Source: CAD feature listing. Evaluate the final solid. Frame: model axes, mm. A direction names the side the tool comes from. Coordinates: 2 decimals unless noted, no trailing zeros. Order: outer loops, then holes, each group sorted by start corner. A loop starts at its lowest first (then second) coordinate and runs counter-clockwise, first axis right, second up.
```python
from build123d import *

# Parameters (mm, degrees)
SKETCH1_W           = 42
SKETCH1_H           = 42
BOSS_EXTRUDE1_DEPTH = 46
CHAMFER1_SIZE       = 5
SKETCH2_R           = 11.5
BOSS_EXTRUDE2_DEPTH = 2
SKETCH3_R           = 2.5
BOSS_EXTRUDE3_DEPTH = 25
SKETCH4_R           = 1.5
CUT_EXTRUDE1_DEPTH  = 5


with BuildPart() as part:
    # Sketch1 → Boss-Extrude1 (new body)
    with BuildSketch(Plane(origin=(0, 0, 0), x_dir=(1, 0, 0), z_dir=(0, 1, 0))):
        Rectangle(SKETCH1_W, SKETCH1_H)
    extrude(amount=BOSS_EXTRUDE1_DEPTH)

    # Chamfer1
    chamfer1_edges = [part.edges().sort_by_distance(p)[0] for p in [
        (21, 23, 21),
        (-21, 23, 21),
        (-21, 23, -21),
        (21, 23, -21),
    ]]
    chamfer(chamfer1_edges, length=CHAMFER1_SIZE)

    # Sketch2 → Boss-Extrude2 (add)
    with BuildSketch(Plane(origin=(0, 46, 0), x_dir=(1, 0, 0), z_dir=(0, 1, 0))):
        with Locations(Location((0, 0, 0), (0, 0, 90))):
            Circle(SKETCH2_R)
    extrude(amount=BOSS_EXTRUDE2_DEPTH)

    # Sketch3 → Boss-Extrude3 (add)
    with BuildSketch(Plane(origin=(0, 46, 0), x_dir=(1, 0, 0), z_dir=(0, 1, 0))):
        with Locations(Location((0, 0, 0), (0, 0, 270))):
            Circle(SKETCH3_R)
    extrude(amount=BOSS_EXTRUDE3_DEPTH)

    # Sketch4 → Cut-Extrude1 (cut)
    with BuildSketch(Plane(origin=(0, 46, 0), x_dir=(1, 0, 0), z_dir=(0, 1, 0))):
        with Locations(Location((-15.909902577, 15.909902577, 0), (0, 0, 270))):
            Circle(SKETCH4_R)
        with Locations(Location((15.909902577, 15.909902577, 0), (0, 0, 270))):
            Circle(SKETCH4_R)
        with Locations(Location((15.909902577, -15.909902577, 0), (0, 0, 270))):
            Circle(SKETCH4_R)
        with Locations(Location((-15.909902577, -15.909902577, 0), (0, 0, 270))):
            Circle(SKETCH4_R)
    extrude(amount=-CUT_EXTRUDE1_DEPTH, mode=Mode.SUBTRACT)


solid = part.part
```
Q1. Pin query (flat end, axial travel): P1, Ø0.9, axis at x = -16.5, z = -15.5, coming from the +Y side; P2, Ø3.5, axis at x = 15.91, z = -15.91, coming from the +Y side. Return the tip coordinate at first contact, or that it passes through.
Solutions:
P1: stops at y = 41
P2: stops at y = 46
Q2. Set-up query: faces 1 (the cylindrical face through (-9.7, 46.99, -6.18)), 2 (the flat face through (-18, 23, 19)). Return all of +Z, -Z, +X, -X, +Y, -Y with unobstructed straight access to the full face (end or side cutting, diameter ignored); none if empty.
Solutions:
face 1: +Y
face 2: +Z, -X, +Y, -Y
Q3. Section query D-D on y = 60. Output: boundary loops of the cut face in (x, z).
Solutions:
outline: circle Ø5 at (0, 0)
Q4. Section query C-C on x = 0. Output: boundary loops of the cut face in (y, z).
Solutions:
outline: (0, -21) - (46, -21) - (46, -11.5) - (48, -11.5) - (48, -2.5) - (71, -2.5) - (71, 2.5) - (48, 2.5) - (48, 11.5) - (46, 11.5) - (46, 21) - (0, 21) - close
Q5. Material intervals for line 1 along Y through (x, z) = (12.5, 4.5); line 2 along Y through (x, z) = (3, 0); line 3 along Z through (x, y) = (0, 65.5), sorted ascending.
Solutions:
line 1: y = 0 to 46
line 2: y = 0 to 48
line 3: z = -2.5 to 2.5
Q6. Section query A-A on y = 11.5. Output: boundary loops of the cut face in (x, z), plus the area to 3 significant figures.
Solutions:
outline: (-21, -16) - (-16, -21) - (16, -21) - (21, -16) - (21, 16) - (16, 21) - (-16, 21) - (-21, 16) - close
area: 1,710 mm2
Q7. Pull-direction query (Z, two-part tool) for faces 3 (the flat face through (19, 23, 18)), 4 (the flat face through (18, 23, -19)), 5 (the flat face through (9, 46, 9)), 6 (the cylindrical face through (16.92, 43.54, 14.8)); classes: pulls with the +Z half, pulls with the -Z half, needs draft (parallel to the pull), parting line crosses it, or undercut.
Solutions:
face 3: pulls with the +Z half
face 4: pulls with the -Z half
face 5: needs draft
face 6: undercut
Q8. Section query B-B on z = 0. Output: boundary loops of the cut face in (x, y).
Solutions:
outline: (-21, 0) - (21, 0) - (21, 46) - (11.5, 46) - (11.5, 48) - (2.5, 48) - (2.5, 71) - (-2.5, 71) - (-2.5, 48) - (-11.5, 48) - (-11.5, 46) - (-21, 46) - close
